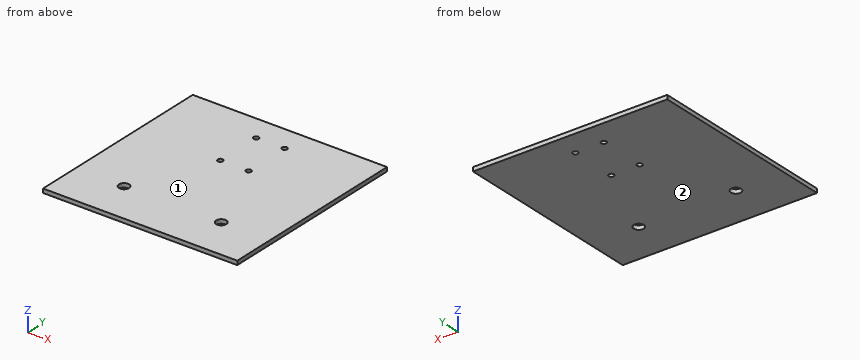
from build123d import *

# Parameters (mm, degrees)
SKETCH1_W               = 152.4
SKETCH1_H               = 152.4
BOSS_EXTRUDE1_DEPTH     = 3.175
CUT_EXTRUDE2_DEPTH      = 2.54
CUT_EXTRUDE2_DEPTH_BACK = 42.418
SKETCH2_R               = 2.032
SKETCH2_5_R             = 4
CUT_EXTRUDE3_DEPTH      = 42.418


with BuildPart() as part:
    # Sketch1 → Boss-Extrude1 (new body)
    with BuildSketch(Plane.XY):
        Rectangle(SKETCH1_W, SKETCH1_H)
    extrude(amount=BOSS_EXTRUDE1_DEPTH)

    # Sketch2 → Cut-Extrude2 (cut, two sides: drawn at the far end of the back side and taken through both)
    with BuildSketch(Plane.XY.offset(3.175).offset(-CUT_EXTRUDE2_DEPTH_BACK)):
        with Locations((-11.1125, 56.3626)):
            Circle(SKETCH2_R)
        with Locations((11.1125, 56.3626)):
            Circle(SKETCH2_R)
        with Locations((11.1125, 19.8374)):
            Circle(SKETCH2_R)
        with Locations((-11.1125, 19.8374)):
            Circle(SKETCH2_R)
    extrude(amount=CUT_EXTRUDE2_DEPTH + CUT_EXTRUDE2_DEPTH_BACK, mode=Mode.SUBTRACT)

    # Sketch2<5> → Cut-Extrude3 (cut)
    with BuildSketch(Plane.XY.offset(3.175)):
        with Locations((-38.1, -43.095115681)):
            Circle(SKETCH2_5_R)
        with Locations((38.1, -43.095115681)):
            Circle(SKETCH2_5_R)
    extrude(amount=-CUT_EXTRUDE3_DEPTH, mode=Mode.SUBTRACT)


solid = part.part
Could you check a few things on this model? Use its own coordinates, in mm. Face numbers are marked on the shaded views. Give positions to 0.01 mm unless a question says otherwise; leave off trailing zeros. Write each loop counter-clockwise with the first axis right and the second up, starting at its lowest first coordinate (ties: lowest second). Pieces come first, ordered by that corner, then holes. Notation, with made-up numbers: (-10, 53.5) -> (46, 53.5) arc R20 cw to (46, 78.5) -> close; hole circle Ø1 at (6.25, 88). An arc over 180 degrees is marked (long way). Answer as a JSON object with one key per item and string values.
Q1. Will this pin go through, and if not, where does the flat tip stop? pin 1 Ø5 at (x, y) = (-38.1, -43.1) entering from +Z.
Taken from the geometry:
{"pin 1": "passes through"}
Q2. Please list where these lines run through material, in increasing order: L1, parallel to Y at x = 11, z = 0.6; L2, parallel to Y at x = 38.1, z = 1.1; L3, parallel to X at y = 18.5, z = 3.
Taken from the geometry:
{"L1": "y = -76.2 to 17.81, 21.87 to 54.33, 58.39 to 76.2", "L2": "y = -76.2 to -47.1, -39.1 to 76.2", "L3": "x = -76.2 to -12.64, -9.58 to 9.58, 12.64 to 76.2"}
Q3. Suppose I cut it at A-A on x = -38.1. Write out the boundary of the cut face in (y, z) (3 decimals).
Taken from the geometry:
{"outline": "(-76.2, 0) -> (-47.095, 0) -> (-47.095, 3.175) -> (-76.2, 3.175) -> close; (-39.095, 0) -> (76.2, 0) -> (76.2, 3.175) -> (-39.095, 3.175) -> close"}
Q4. We'd pull the mould along Z, two halves only. Please class the marked faces 1 and 2: released by +Z, released by -Z, zero draft, split by the parting line, or undercut.
Taken from the geometry:
{"face 1": "released by +Z", "face 2": "released by -Z"}
